from build123d import *

# Parameters (mm, degrees)
F1_DEPTH  = 2.5
F2_T      = -2
F5_SIZE   = 1
F6_W      = 75
F6_H      = 5
F6_R      = 2
F7_DEPTH  = 37.501
F8_W      = 1
F8_H      = 7.945
F9_DEPTH  = 6
F12_R     = 5
F13_DEPTH = 5
F15_D     = 5.5


with BuildPart() as f1:
    # F0 (on Front) → F1 (new body, symmetric)
    with BuildSketch(Plane.XZ):
        with BuildLine():
            Line((0, 10), (0, 0))
            Line((0, 0), (70, 0))
            Line((70, 0), (70, 10))
            Line((70, 10), (50, 10))
            ThreePointArc((50, 10), (46.4644660941, 11.4644660941), (45, 15))
            Line((45, 15), (45, 25))
            Line((45, 25), (35, 25))
            Line((35, 25), (35, 15))
            ThreePointArc((35, 15), (33.5355339059, 11.4644660941), (30, 10))
            Line((30, 10), (0, 10))
        make_face()
    extrude(amount=F1_DEPTH, both=True)

    # F2
    f2_openings = [f1.faces().sort_by_distance(p)[0] for p in [
        (35.933685, -2.5, 7.254637),
    ]]
    offset(amount=F2_T, openings=f2_openings)

    # F3 (on Front) → F4 (revolve)
    with BuildSketch(Plane.XZ):
        Polygon((40, 25), (40, 37.5), (37, 37.5), (37, 35.5), (37.5, 35.5), (37.5, 27), (37, 27), (37, 25), align=None)
    revolve(axis=Axis((40, 0, 31.25), (0, 0, 1)))

    # F5
    f5_edges = [f1.edges().sort_by_distance(p)[0] for p in [
        (43, 0, 37.5),
    ]]
    chamfer(f5_edges, length=F5_SIZE)

    # F6 (on face) → F7 (intersect, through all)
    with BuildSketch(Plane.XY.offset(37.5)):
        with Locations((35.3798213182, 0)):
            Rectangle(F6_W, F6_H)
        with Locations((40, 0)):
            Circle(F6_R, mode=Mode.SUBTRACT)
        with Locations((40, 0)):
            Circle(F6_R)
    extrude(amount=-F7_DEPTH, mode=Mode.INTERSECT)

    # F8 (on face) → F9 (cut)
    with BuildSketch(Plane.XY.offset(37.5)):
        with Locations((40, -0.2165465654)):
            Rectangle(F8_W, F8_H)
    extrude(amount=-F9_DEPTH, mode=Mode.SUBTRACT)

    # F10: F1 across plane


with BuildPart() as f1_1:
    add(f1.part)
    add(f1.part.mirror(Plane.XY))

    # F11: F1 across plane


with BuildPart() as f1_2:
    add(f1_1.part)
    add(f1_1.part.mirror(Plane.YZ))

    # F12 (on face) → F13 (join, through all)
    with BuildSketch(Plane.XZ.offset(2.5)):
        with Locations((-40, 0)):
            Circle(F12_R)
        with Locations((-15, 0)):
            Circle(F12_R)
    extrude(amount=-F13_DEPTH)

    # F15 (through all)
    with Locations(Plane.XZ.offset(2.5)):
        with Locations((-40, 0), (-15, 0)):
            Hole(F15_D / 2)


solid = f1_2.part
Build history of the part. All positions in model axes, mm. A direction names the side the tool comes from. Coordinates: 2 decimals unless noted, no trailing zeros. Write each loop counter-clockwise with the first axis right and the second up, starting at its lowest first coordinate (ties: lowest second). Pieces come first, ordered by that corner, then holes.
(1) Pin check, flat tips, straight feed: pin 1 Ø1.5 at (x, y) = (14.5, -1) entering from -Z; pin 2 Ø3 at (y, z) = (0, 18.5) entering from -X; pin 3 Ø0.9 at (x, y) = (-51.5, -0.5) entering from +Z. Stop position of each tip, or through.
(2) Cut at B-B on z = 0. List the corners of the cut face in (x, y), and give its area (3 significant figures).
(3) Drill centre lines: line 1 (Z direction, x = -40, y = -0.7); line 2 (Z direction, x = -15, y = -1.4); line 3 (X direction, y = 1.9, z = -23). Where is each one in solid material? Low to high.
(4) 3-axis set-ups, long thin cutter, end or side, ignore diameter. For faces 1 (the cylindrical face through (38.85, 2.22, -31.19)), 2 (the flat face through (-37, -1, 19)), 3 (the flat face through (-35, 0, -20)), 4 (the flat face through (35, 0, 20)): which of +Z, -Z, +X, -X, +Y, -Y reach the whole face in a straight line?
(5) Cut at C-C on x = -15. List the corners of the cut face in (y, z), and give its area (3 significant figures).
(6) Mould opens along Z. For faces 5 (the flat face through (-6, -1, -2)), 6 (the flat face through (-42.7, -0.2, -35.5)), 7 (the conical face through (-37.8, 0, 37.3)), 8 (the flat face through (70, 0, 0)) say: pulls with the +Z half, pulls with the -Z half, needs draft (parallel to the pull), parting line crosses it, or undercut.
(7) Cut at D-D on x = 18. List the corners of the cut face in (y, z).
(8) Cut at A-A on z = 16.5. List the corners of the cut face in (x, y).
Working result:
1. pin 1: stops at z = -10
1. pin 2: stops at x = -45
1. pin 3: stops at z = 10
2. outline: (-70, -2.5) - (-42.75, -2.5) - (-42.75, 2.5) - (-70, 2.5) - close; (-37.25, -2.5) - (-17.75, -2.5) - (-17.75, 2.5) - (-37.25, 2.5) - close; (-12.25, -2.5) - (70, -2.5) - (70, 2.5) - (-12.25, 2.5) - close
2. area: 645 mm2
3. line 1: z = -31.5 to -23, -5 to -2.75, 2.75 to 5, 23 to 31.5
3. line 2: z = -10 to -8, -5 to -2.75, 2.75 to 5, 8 to 10
3. line 3: x = -45 to -35, 35 to 45
4. face 1: none
4. face 2: -Y
4. face 3: -Z, +Y, -Y
4. face 4: +Z, +Y, -Y
5. outline: (-2.5, -10) - (2.5, -10) - (2.5, -2.75) - (-2.5, -2.75) - (-2.5, -5) - (0.5, -5) - (0.5, -8) - (-2.5, -8) - close; (-2.5, 2.75) - (2.5, 2.75) - (2.5, 10) - (-2.5, 10) - (-2.5, 8) - (0.5, 8) - (0.5, 5) - (-2.5, 5) - close
5. area: 54.5 mm2
6. face 5: undercut
6. face 6: undercut
6. face 7: pulls with the +Z half
6. face 8: needs draft
7. outline: (-2.5, -10) - (2.5, -10) - (2.5, 10) - (-2.5, 10) - (-2.5, 8) - (0.5, 8) - (0.5, 2) - (-2.5, 2) - (-2.5, -2) - (0.5, -2) - (0.5, -8) - (-2.5, -8) - close
8. outline: (-45, -2.5) - (-43, -2.5) - (-43, 0.5) - (-37, 0.5) - (-37, -2.5) - (-35, -2.5) - (-35, 2.5) - (-45, 2.5) - close; (35, -2.5) - (37, -2.5) - (37, 0.5) - (43, 0.5) - (43, -2.5) - (45, -2.5) - (45, 2.5) - (35, 2.5) - close
